from build123d import *

# Parameters (mm, degrees)
SKETCH1_W           = 350
SKETCH1_H           = 350
BOSS_EXTRUDE1_DEPTH = 150
BOSS_EXTRUDE2_DEPTH = 175
BOSS_EXTRUDE3_DEPTH = 175


with BuildPart() as part:
    # Sketch1 → Boss-Extrude1 (new body)
    with BuildSketch(Plane(origin=(0, 0, 0), x_dir=(1, 0, 0), z_dir=(0, 1, 0))):
        Rectangle(SKETCH1_W, SKETCH1_H)
    extrude(amount=BOSS_EXTRUDE1_DEPTH)

    # Sketch2 → Boss-Extrude2 (add, symmetric)
    with BuildSketch(Plane(origin=(0, 0, 0), x_dir=(0, 0, -1), z_dir=(1, 0, 0))):
        Polygon((-175, 150), (-175, 0), (-558.723859044, 0), align=None)
    extrude(amount=BOSS_EXTRUDE2_DEPTH, both=True)

    # Sketch3 → Boss-Extrude3 (add, symmetric)
    with BuildSketch(Plane.XY):
        Polygon((-175, 150), (-558.723859044, 0), (-175, 0), align=None)
        Polygon((175, 150), (175, 0), (558.723859044, 0), align=None)
    extrude(amount=BOSS_EXTRUDE3_DEPTH, both=True)


solid = part.part
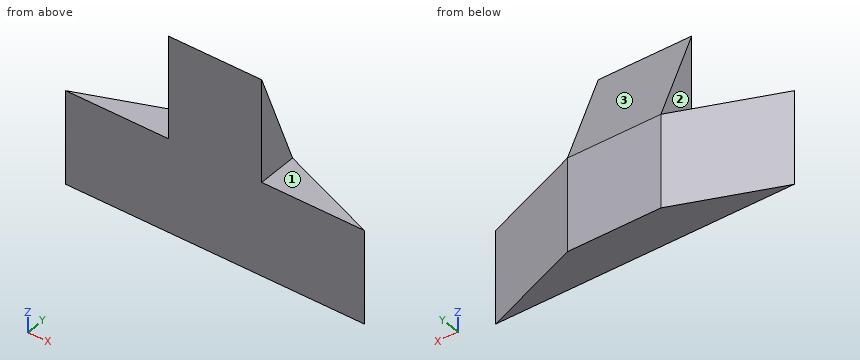
Read the model definition and answer for the solid it produces. Units are mm, in the model's axes. Face numbers are marked on the shaded views. A direction names the side the tool comes from. Round coordinates to 2 decimals unless told otherwise and drop trailing zeros. Write each loop counter-clockwise with the first axis right and the second up, starting at its lowest first coordinate (ties: lowest second). Pieces come first, ordered by that corner, then holes.
1. Which of the six approach directions +Z, -Z, +X, -X, +Y, -Y give full straight-line access (tool end or side, diameter ignored) to the marked faces 1, 2 and 3?
2. Straight lines are drawn through the part: L1, parallel to X at y = 47.5, z = 191.5; L2, parallel to Y at x = 225.5, z = 162. For each, find the intervals that lie inside material, in ascending order.
3. The part is cut by section B-B, the plane z = 16. Determine the outline of the cut face in (x, y), then the cut area to 3 significant figures.
4. Given pin 1 Ø1.5 at (y, z) = (77, 192) entering from -X; pin 2 Ø5 at (y, z) = (72, 259.5) entering from +X, each flat-ended and moving along its own axis, determine where each tip first touches the part or whether it passes through.
5. The part is cut by section C-C, the plane x = 31.5. Determine the outline of the cut face in (y, z), then the cut area to 3 significant figures.
6. The part is cut by section D-D, the plane y = 129.5. Determine the outline of the cut face in (x, z).
7. The part is cut by section A-A, the plane y = 76.5. Determine the outline of the cut face in (x, z).
Values:
1. face 1: +Z, +X, +Y, -Y
1. face 2: +Z, -X, +Y, -Y
1. face 3: +Z, +X, -X, +Y
2. L1: x = -175 to 175
2. L2: y = 0 to 130.26
3. outline: (-558.72, 0) - (558.72, 0) - (175, 150) - (-175, 150) - close
3. area: 110,000 mm2
4. pin 1: stops at x = -175
4. pin 2: stops at x = 175
5. outline: (0, -175) - (150, -175) - (150, 175) - (0, 558.72) - close
5. area: 81,300 mm2
6. outline: (-227.44, -175) - (227.44, -175) - (227.44, 175) - (175, 175) - (175, 227.44) - (-175, 227.44) - (-175, 175) - (-227.44, 175) - close
7. outline: (-363.02, -175) - (363.02, -175) - (363.02, 175) - (175, 175) - (175, 363.02) - (-175, 363.02) - (-175, 175) - (-363.02, 175) - close
